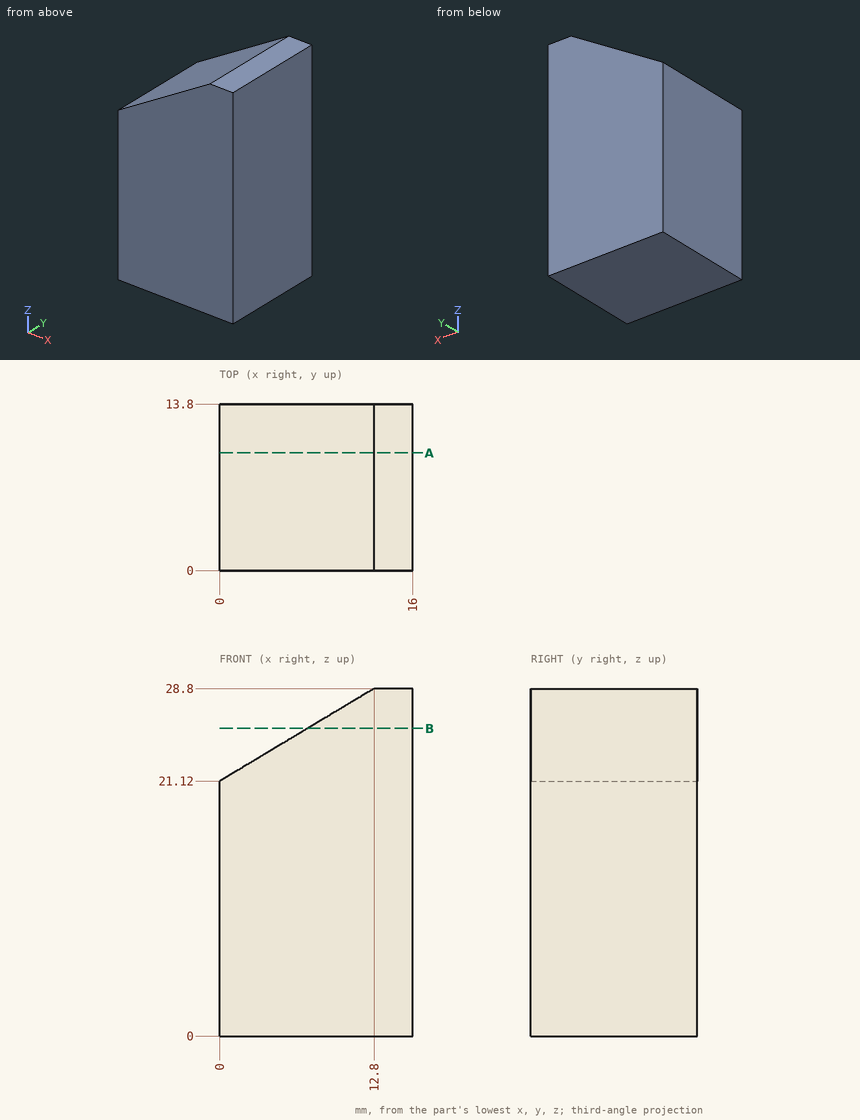
Input: dimensioned drawing with shaded views. Units: mm. Origin: part minimum x, y, z. Coordinates: 2 decimals unless noted, no trailing zeros. Loops run counter-clockwise (first coordinate to the right, second up) from the corner with the lowest first, then second, coordinate; pieces in that order, holes last.
Q1. Section B-B, the plane z = 25.5. Return the cut outline in (x, y), and give its area (3 significant figures).
Results are:
outline: (7.3, 0) - (16, 0) - (16, 13.8) - (7.3, 13.8) - close
area: 120 mm2
Q2. Contact query for flat-ended pins moving along their axis: pin 1 (4 mm diameter, centred on x = 5.5, y = 2, fed in from +Z); pin 2 (4 mm diameter, centred on x = 2.5, y = 5.5, fed in from +Z). Output: stop coordinate, or through.
Results are:
pin 1: stops at z = 25.62
pin 2: stops at z = 23.82
Q3. Section A-A, the plane y = 9.75. Return the cut outline in (x, z).
Results are:
outline: (0, 0) - (16, 0) - (16, 28.8) - (12.8, 28.8) - (0, 21.12) - close
Q4. Line query: line 1 along Z through (x, y) = (5, 2.5); line 2 along Z through (x, y) = (11, 6.25); line 3 along X through (y, z) = (4.5, 21.25). Output: solid intervals per line, ascending.
Results are:
line 1: z = 0 to 24.12
line 2: z = 0 to 27.72
line 3: x = 0.22 to 16
